Work out the finished part from the listing and answer in its coordinate system (mm). A direction names the side the tool comes from. Round coordinates to 2 decimals unless told otherwise and drop trailing zeros. Loops run counter-clockwise (first coordinate to the right, second up) from the corner with the lowest first, then second, coordinate; pieces in that order, holes last. Notation, with made-up numbers: (79.25, 38) -> (127.25, 38) arc R17 ccw to (127.25, 69) -> close; hole circle Ø2 at (-15.5, 23.5). An arc over 180 degrees is marked (long way). Write item = value, one per line. Start each with the question number.
```python
from build123d import *

# Parameters (mm, degrees)
F0_W     = 70
F0_H     = 40
F1_DEPTH = 10
F2_W     = 39
F2_H     = 29
F3_DEPTH = 15
F4_R     = 5
F5_DEPTH = 25


with BuildPart() as f1:
    # F0 (on Right) → F1 (new body)
    with BuildSketch(Plane.YZ):
        with Locations((35, 20)):
            Rectangle(F0_W, F0_H)
    extrude(amount=F1_DEPTH)

    # F2 (on face) → F3 (join)
    with BuildSketch(Plane.YZ.offset(10)):
        with Locations((35, 20)):
            Rectangle(F2_W, F2_H)
    extrude(amount=-F3_DEPTH)

    # F4 (on face) → F5 (cut)
    with BuildSketch(Plane.YZ.offset(10)):
        with Locations((35, 20.140665)):
            Circle(F4_R)
    extrude(amount=-F5_DEPTH, mode=Mode.SUBTRACT)


solid = f1.part
```
Item 1: A tool of negligible diameter and unlimited length cuts with its end or side. For faces 4 (the flat face through (5, 35, 0)), 5 (the flat face through (-2, 15.5, 20)), 6 (the flat face through (-2, 54.5, 20)), 7 (the flat face through (-2, 35, 34.5)), 8 (the flat face through (5, 0, 20)), from which of +Z, -Z, +X, -X, +Y, -Y can it reach the whole face along a straight path? Write none if from no direction.
Item 2: Section D-D (x = 5.75) is taken. Determine the outline of the cut face in (y, z).
Item 3: Find the intervals of material crossed by line 1 along Z through (x, y) = (7, 35); line 2 along Z through (x, y) = (-0.5, 35); line 3 along Y through (x, z) = (4.25, 20), in increasing order. Write a range as [from, to].
Item 4: Section C-C (y = 18.5) is taken. Determine the outline of the cut face in (x, z).
Item 5: Section A-A (y = 35) is taken. Determine the outline of the cut face in (x, z), then the cut area to 3 significant figures.
Item 6: Flat-ended cylindrical pins translate along their axes: pin 1 (1.5 mm diameter, centred on x = -3.5, y = 35.5, fed in from +Z); pin 2 (4 mm diameter, centred on x = -3, y = 30, fed in from -Z); pin 3 (1.5 mm diameter, centred on x = -2.5, z = 20.5, fed in from -Y); pin 4 (8 mm diameter, centred on y = 35, z = 20.14, fed in from +X) (1 decimal). Find the tip coordinate at first contact, or state that the pin passes through.
Item 7: Section B-B (z = 33.5) is taken. Determine the outline of the cut face in (x, y).
Item 8: The mould has two halves that part along Y. Classify faces 1 (the cylindrical face through (3, 30, 20)), 2 (the flat face through (-2, 35, 5.5)), 3 (the flat face through (5, 70, 20)): pulls with the +Y half, pulls with the -Y half, needs draft (parallel to the pull), parting line crosses it, or undercut.
Worked answers:
q1.face_4 = -Z, +X, -X, +Y, -Y
q1.face_5 = +Z, -Z, -X, -Y
q1.face_6 = +Z, -Z, -X, +Y
q1.face_7 = +Z, -X, +Y, -Y
q1.face_8 = +Z, -Z, +X, -X, -Y
q2.outline = (0, 0) -> (70, 0) -> (70, 40) -> (0, 40) -> close; hole circle Ø10 at (35, 20.14)
q3.line_1 = [0, 15.14], [25.14, 40]
q3.line_2 = [5.5, 15.14], [25.14, 34.5]
q3.line_3 = [0, 30], [40, 70]
q4.outline = (-5, 5.5) -> (0, 5.5) -> (0, 0) -> (10, 0) -> (10, 40) -> (0, 40) -> (0, 34.5) -> (-5, 34.5) -> close
q5.outline = (-5, 5.5) -> (0, 5.5) -> (0, 0) -> (10, 0) -> (10, 15.14) -> (-5, 15.14) -> close; (-5, 25.14) -> (10, 25.14) -> (10, 40) -> (0, 40) -> (0, 34.5) -> (-5, 34.5) -> close
q5.area = 395 mm2
q6.pin_1 = 34.5
q6.pin_2 = 5.5
q6.pin_3 = 15.5
q6.pin_4 = through
q7.outline = (-5, 15.5) -> (0, 15.5) -> (0, 0) -> (10, 0) -> (10, 70) -> (0, 70) -> (0, 54.5) -> (-5, 54.5) -> close
q8.face_1 = undercut
q8.face_2 = needs draft
q8.face_3 = pulls with the +Y half
